```python
from build123d import *

# Parameters (mm, degrees)
F0_R       = 12.835001
F1_DEPTH   = 12.7
F2_R       = 1.905
F1_FACE_W  = 37.6999124221
F1_FACE_H  = 12.7
F1_FACE1_W = 13.7613505735
F1_FACE1_H = 12.7
F3_DEPTH   = 0.254
F4_DEPTH   = 4.7498


with BuildPart() as f1:
    # F0 (on Top) → F1 (new body)
    with BuildSketch(Plane.XY):
        with BuildLine():
            Line((-33.4334959418, 33.5081874669), (-30.4082068312, 35.4751199209))
            ThreePointArc((-30.4082068312, 35.4751199209), (-41.4944322517, 64.6897953257), (-43.5214952555, 33.5081874669))
            Line((-43.5214952555, 33.5081874669), (-43.5214952555, 24.2223944372))
            Line((-43.5214952555, 24.2223944372), (-57.282845829, 24.2223944372))
            Line((-57.282845829, 24.2223944372), (-57.282845829, 21.0543349588))
            Line((-57.282845829, 21.0543349588), (-19.5829334069, 21.0543349588))
            Line((-19.5829334069, 21.0543349588), (-19.5829334069, 24.2223944372))
            Line((-19.5829334069, 24.2223944372), (-33.4334959418, 24.2223944372))
            Line((-33.4334959418, 24.2223944372), (-33.4334959418, 33.5081874669))
        make_face()
        with Locations((-39.122876168, 48.8789326412)):
            Circle(F0_R, mode=Mode.SUBTRACT)
    extrude(amount=F1_DEPTH)

    # F2 (on face) + F1_face (on face) + F1_face1 (on face) → F3 (join)
    with BuildSketch(Plane.XZ.offset(-21.0543349588)):
        with Locations((-51.7907068133, 6.3078426756)):
            Circle(F2_R)
    with BuildSketch(Plane(origin=(-38.432889618, 21.0543349588, 6.35), x_dir=(1, 0, 0), z_dir=(0, -1, 0))):
        Rectangle(F1_FACE_W, F1_FACE_H)
    with BuildSketch(Plane(origin=(-50.4021705423, 24.2223944372, 6.35), x_dir=(-1, 0, 0), z_dir=(0, 1, 0))):
        Rectangle(F1_FACE1_W, F1_FACE1_H)
    extrude(amount=-F3_DEPTH, dir=(0, -1, 0))

    # F2 (on face) → F4 (cut)
    with BuildSketch(Plane.XZ.offset(-21.0543349588)):
        with Locations((-24.7001815587, 6.4406394958)):
            Circle(F2_R)
        with Locations((-51.7907068133, 6.3078426756)):
            Circle(F2_R)
    extrude(amount=-F4_DEPTH, mode=Mode.SUBTRACT)


solid = f1.part
```
Could you check a few things on this model? Use its own coordinates, in mm. A direction names the side the tool comes from. Coordinates: 2 decimals unless noted, no trailing zeros. Loops run counter-clockwise (first coordinate to the right, second up) from the corner with the lowest first, then second, coordinate; pieces in that order, holes last.
1) Please list where these lines run through material, in increasing order: line 1 along Y through (x, z) = (-32.5, 8.75); line 2 along Y through (x, z) = (-48.5, 11); line 3 along X through (y, z) = (46, 11).
Reported:
line 1: y = 21.05 to 24.22, 34.12 to 37.88, 59.87 to 63.43
line 2: y = 21.05 to 24.48, 35.93 to 40.11, 57.64 to 61.83
line 3: x = -54.85 to -51.63, -26.61 to -23.4
2) Imagine slicing it at C-C (x = -38.5). List the corners of the cut face in (y, z) for me.
Reported:
outline: (21.05, 0) - (36.06, 0) - (36.06, 12.7) - (21.05, 12.7) - close; (61.7, 0) - (64.85, 0) - (64.85, 12.7) - (61.7, 12.7) - close
3) Thinking about a two-plate mould opening in Z: for faces 1 (the face through (-39, 35, 0)), 2 (the face through (-50.767, 22.741, 7.914)), 3 (the face through (-19.583, 23, 6)), 4 (the face through (-23.82, 22.62, 4.75)), which applies, released by +Z, released by -Z, zero draft, split by the parting line, or undercut?
Reported:
face 1: released by -Z
face 2: undercut
face 3: zero draft
face 4: undercut
4) Will these pins go through, and if not, where does the flat tip stop? pin 1 Ø3 at (y, z) = (29.5, 4.5) entering from +X; pin 2 Ø1 at (y, z) = (52.5, 2) entering from +X; pin 3 Ø7 at (y, z) = (29, 7.5) entering from -X; pin 4 Ø6 at (x, y) = (-29, 40) entering from -Z.
Reported:
pin 1: stops at x = -33.43
pin 2: stops at x = -23.44
pin 3: stops at x = -43.52
pin 4: stops at z = 0
5) Imagine slicing it at B-B (y = 46.5). List the corners of the cut face in (x, z) for me.
Reported:
outline: (-54.93, 0) - (-51.74, 0) - (-51.74, 12.7) - (-54.93, 12.7) - close; (-26.51, 0) - (-23.31, 0) - (-23.31, 12.7) - (-26.51, 12.7) - close
6) Which directions (+Z, -Z, +X, -X, +Y, -Y) give clear straight access to the entire face, cutting with the end or side of a thin tool? Please do faces 5 (the face through (-39, 35, 12.7)), 6 (the face through (-31.94, 34.48, 6.26)), 7 (the face through (-50, 24.476, 5)).
Reported:
face 5: +Z, +X, -X, +Y, -Y
face 6: +Z, -Z, +X
face 7: +Z, -Z, -X
7) Imagine slicing it at D-D (z = 5.25). List the corners of the cut face in (x, y) for me (1 decimal), and give its area (3 significant figures).
Reported:
outline: (-57.3, 21.1) - (-53.4, 21.1) - (-53.4, 24.5) - (-57.3, 24.5) - close; (-50.2, 21.1) - (-26.2, 21.1) - (-26.2, 24.2) - (-33.4, 24.2) - (-33.4, 33.5) - (-30.4, 35.5) arc R16 ccw (long way) to (-43.5, 33.5) - (-43.5, 24.5) - (-50.2, 24.5) - close; (-23.2, 21.1) - (-19.6, 21.1) - (-19.6, 24.2) - (-23.2, 24.2) - close; hole circle Ø25.7 at (-39.1, 48.9)
area: 479 mm2
8) Imagine slicing it at A-A (z = 7.5). List the corners of the cut face in (x, y) for me (1 decimal), and give its area (3 significant figures).
Reported:
outline: (-57.3, 21.1) - (-53.3, 21.1) - (-53.3, 24.5) - (-57.3, 24.5) - close; (-50.3, 21.1) - (-26.3, 21.1) - (-26.3, 24.2) - (-33.4, 24.2) - (-33.4, 33.5) - (-30.4, 35.5) arc R16 ccw (long way) to (-43.5, 33.5) - (-43.5, 24.5) - (-50.3, 24.5) - close; (-23.1, 21.1) - (-19.6, 21.1) - (-19.6, 24.2) - (-23.1, 24.2) - close; hole circle Ø25.7 at (-39.1, 48.9)
area: 479 mm2
